Here's how the part is built. I have some questions about the finished solid (model axes, mm). A direction names the side the tool comes from. Round coordinates to 2 decimals unless told otherwise and drop trailing zeros. Loops run counter-clockwise (first coordinate to the right, second up) from the corner with the lowest first, then second, coordinate; pieces in that order, holes last. Notation, with made-up numbers: M 62,-22.75 L 79,-22.75 A25 cw 79,-4.75 Z; hole C 2.5,-34 d10. An arc over 180 degrees is marked long. Write item = value, one per line. Start each with the question number.
from build123d import *

# Parameters (mm, degrees)
F2_R    = 1.27
F3_SIZE = 1.27


with BuildPart() as f1:
    # F0 (on Front) → F1 (revolve)
    with BuildSketch(Plane.XZ):
        Polygon((7.14375, 19.05), (0, 19.05), (0, -12.7), (7.14375, -12.7), (7.14375, 0), (19.05, 0), (19.05, 6.35), (7.14375, 6.35), align=None)
    revolve(axis=Axis((0, 0, 3.175), (0, 0, -1)))

    # F2
    f2_edges = [f1.edges().sort_by_distance(p)[0] for p in [
        (-19.05, 0, 6.35),
        (-19.05, 0, 0),
    ]]
    fillet(f2_edges, radius=F2_R)

    # F3
    f3_edges = [f1.edges().sort_by_distance(p)[0] for p in [
        (-7.14375, 0, 19.05),
        (-7.14375, 0, -12.7),
    ]]
    chamfer(f3_edges, length=F3_SIZE)


solid = f1.part
Item 1: Will these pins go through, and if not, where does the flat tip stop? pin 1 Ø1 at (y, z) = (14.5, 2) entering from -X; pin 2 Ø10 at (x, z) = (5.5, 15.5) entering from -Y; pin 3 Ø8 at (x, z) = (-8.5, 6) entering from -Y.
Item 2: I want a section at A-A, the plane y = 0. List the corners of the cut face in (x, z) for me.
Item 3: Please list where these lines run through material, in increasing order: line 1 (Z direction, x = -9.5, y = -13); line 2 (Z direction, x = 16.5, y = 8.5); line 3 (X direction, y = 2, z = 8.5). Write a range as [from, to].
Item 4: I want a section at C-C, the plane z = 7. List the corners of the cut face in (x, y) for me, then the cut area to 3 significant figures.
Item 5: For faces 1 (the flat face through (0, 8, 6.35)), 2 (the flat face through (0, 0, 19.05)), 3 (the cylindrical face through (-7.137, -0.314, -5.635)), which set-ups out of +Z, -Z, +X, -X, +Y, -Y let a thin tool reach every point of the face, with its end or its side?
Worked out:
q1.pin_1 = -12.92
q1.pin_2 = -7.13
q1.pin_3 = -18.49
q2.outline = M -19.05,1.27 A1.27 ccw -17.78,0 L -7.14,0 L -7.14,-11.43 L -5.87,-12.7 L 5.87,-12.7 L 7.14,-11.43 L 7.14,0 L 17.78,0 A1.27 ccw 19.05,1.27 L 19.05,5.08 A1.27 ccw 17.78,6.35 L 7.14,6.35 L 7.14,17.78 L 5.87,19.05 L -5.87,19.05 L -7.14,17.78 L -7.14,6.35 L -17.78,6.35 A1.27 ccw -19.05,5.08 Z
q3.line_1 = [0, 6.35]
q3.line_2 = [0.27, 6.08]
q3.line_3 = [-6.86, 6.86]
q4.outline = C 0,0 d14.29
q4.area = 160 mm2
q5.face_1 = +Z
q5.face_2 = +Z, +X, -X, +Y, -Y
q5.face_3 = -Z
